Geometry check sheet. Reference: the model listing, model coordinates, mm. Face numbers are marked on the shaded views. Give positions to 0.01 mm unless a question says otherwise; leave off trailing zeros. Loops run counter-clockwise (first coordinate to the right, second up) from the corner with the lowest first, then second, coordinate; pieces in that order, holes last. Notation, with made-up numbers: (-7.75, 13) - (8.25, 13) arc R32 cw to (8.25, 48) - close; hole circle Ø3 at (46.25, 53.25). An arc over 180 degrees is marked (long way). Use a Markdown table: item, result. Add a question column.
1. Cross-section at A-A on z = 0. Enter the section's corners in (x, y), and give its area (3 significant figures).
2. Cross-section at B-B on x = 20. Enter the section's corners in (y, z), and give its area (3 significant figures).
3. Draft check along Z on the marked faces 1, 2, 3 and 4. Enter one of: pulls with the +Z half, pulls with the -Z half, needs draft (parallel to the pull), parting line crosses it, or undercut.
4. Cross-section at C-C on y = 3. Enter the section's corners in (x, z), and give its area (3 significant figures).
5. Depth check by flat-ended pin: P1, Ø9, axis at x = 0, z = 0, coming from the -Y side. Enter the tip coordinate at first touch or a pass-through.
6. Material ranges on L1, parallel to X at y = 6.25, z = 0; L2, parallel to X at y = 7.5, z = -20; L3, parallel to Z at x = -1, y = 6.25, recorded low to high.
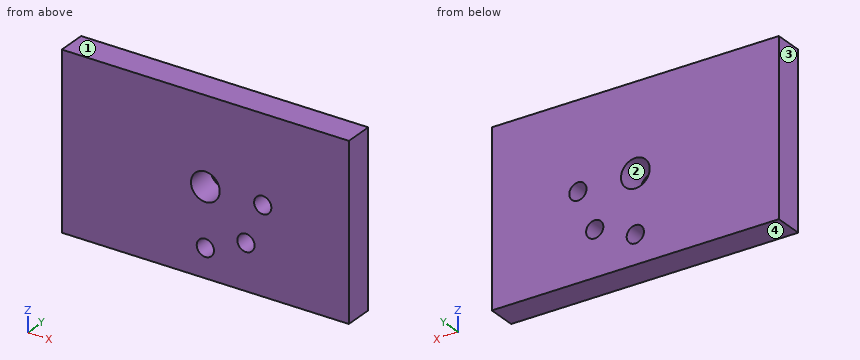
from build123d import *

# Parameters (mm, degrees)
SKETCH_1_W               = 100
SKETCH_1_H               = 60
EXTRUDE_1_DEPTH          = 10
SKETCH_2_R               = 5
CUT_EXTRUDE_1_DEPTH      = 20
SKETCH_3_R               = 3
CUT_EXTRUDE_2_DEPTH      = 20
PATTERN_CIRCULAR_1_COUNT = 3
PATTERN_CIRCULAR_1_ANGLE = 90


with BuildPart() as part:
    # 草图1 → 凸台-拉伸1 (new body)
    with BuildSketch(Plane(origin=(0, 0, 0), x_dir=(1, 0, 0), z_dir=(0, 1, 0))):
        Rectangle(SKETCH_1_W, SKETCH_1_H)
    extrude(amount=EXTRUDE_1_DEPTH)

    # 草图2 → 切除-拉伸1 (cut)
    with BuildSketch(Plane(origin=(0, 0, 0), x_dir=(1, 0, 0), z_dir=(0, 1, 0))):
        with Locations(Location((0, 0, 0), (0, 0, 90))):
            Circle(SKETCH_2_R)
    extrude(amount=CUT_EXTRUDE_1_DEPTH, mode=Mode.SUBTRACT)

    # 草图3 → 切除-拉伸2 (cut)
    with BuildSketch(Plane(origin=(0, 0, 0), x_dir=(1, 0, 0), z_dir=(0, 1, 0))):
        with Locations(Location((20, 0, 0), (0, 0, 90))):
            Circle(SKETCH_3_R)
    cut_extrude_2 = extrude(amount=CUT_EXTRUDE_2_DEPTH, mode=Mode.SUBTRACT)

    # 阵列(圆周)1: 切除-拉伸2 ×3 about axis
    pattern_circular_1_axis = Axis((0, 0, 0), (0, 1, 0))
    for i in range(1, PATTERN_CIRCULAR_1_COUNT):
        add(cut_extrude_2.rotate(pattern_circular_1_axis, i * PATTERN_CIRCULAR_1_ANGLE / (PATTERN_CIRCULAR_1_COUNT - 1)), mode=Mode.SUBTRACT)


solid = part.part
Values found:
| question | item | result |
|---|---|---|
| 1 | outline | (-50, 0) - (-5, 0) - (-5, 10) - (-50, 10) - close; (5, 0) - (17, 0) - (17, 10) - (5, 10) - close; (23, 0) - (50, 0) - (50, 10) - (23, 10) - close |
| 1 | area | 840 mm2 |
| 2 | outline | (0, -30) - (10, -30) - (10, -3) - (0, -3) - close; (0, 3) - (10, 3) - (10, 30) - (0, 30) - close |
| 2 | area | 540 mm2 |
| 3 | face 1 | pulls with the +Z half |
| 3 | face 2 | undercut |
| 3 | face 3 | needs draft |
| 3 | face 4 | pulls with the -Z half |
| 4 | outline | (-50, -30) - (50, -30) - (50, 30) - (-50, 30) - close; hole circle Ø10 at (0, 0); hole circle Ø6 at (0, -20); hole circle Ø6 at (14.14, -14.14); hole circle Ø6 at (20, 0) |
| 4 | area | 5,840 mm2 |
| 5 | P1 | passes through |
| 6 | L1 | x = -50 to -5, 5 to 17, 23 to 50 |
| 6 | L2 | x = -50 to -3, 3 to 50 |
| 6 | L3 | z = -30 to -22.83, -17.17 to -4.9, 4.9 to 30 |
